Source: CAD feature listing. Evaluate the final solid. Frame: model axes, mm. A direction names the side the tool comes from. Round coordinates to 2 decimals unless told otherwise and drop trailing zeros. Write each loop counter-clockwise with the first axis right and the second up, starting at its lowest first coordinate (ties: lowest second). Pieces come first, ordered by that corner, then holes.
Autodesk Fusion 360 part; units mm, degrees
sketch "Sketch1" plane through (0, 0, 0) normal (0, 1, 0) x (1, 0, 0)
  line L0 (25, 18) -> (-25, 18) construction
  line L1 (-25, 18) -> (-25, -18) construction
  line L2 (-25, -18) -> (25, -18) construction
  line L3 (25, -18) -> (25, 18) construction
  line L4 (25, 18) -> (-25, -18) construction
  line L5 (-25, 18) -> (25, -18) construction
  arc A0 (25, 18) -> (-25, 18) centre (0, -84.6667) ccw
  arc A1 (-25, -18) -> (25, -18) centre (0, 84.6667) ccw
  arc A2 (25, -18) -> (25, 18) centre (-27.5, 0) ccw
  arc A3 (-25, 18) -> (-25, -18) centre (27.5, 0) ccw
  arc A4 (-23.0621, -15.8893) -> (23.0621, -15.8893) centre (0, 84.6667) ccw
  arc A5 (23.0621, -15.8893) -> (23.0621, 15.8893) centre (-27.5, 0) ccw
  arc A6 (23.0621, 15.8893) -> (-23.0621, 15.8893) centre (0, -84.6667) ccw
  arc A7 (-23.0621, 15.8893) -> (-23.0621, -15.8893) centre (27.5, 0) ccw
  dimension "d1" = 50
  dimension "d2" = 36
  dimension "d3" = 42
  dimension "d4" = 56
  dimension "d5" = 2.5
extrude "Extrude1" add sketch "Sketch1" along normal blind 170
sketch "Sketch3" plane through (0, 0, 0) normal (0, -1, 0) x (-1, 0, 0)
  arc A0 (23.0621, -15.8893) -> (23.0621, 15.8893) centre (-27.5, 0) ccw
  arc A1 (-23.0621, -15.8893) -> (23.0621, -15.8893) centre (0, 84.6667) ccw
  arc A2 (-23.0621, 15.8893) -> (-23.0621, -15.8893) centre (27.5, 0) ccw
  arc A3 (23.0621, 15.8893) -> (-23.0621, 15.8893) centre (0, -84.6667) ccw
  arc A4 (25, -18) -> (25, 18) centre (-27.5, 0) ccw
  arc A5 (25, 18) -> (-25, 18) centre (0, -84.6667) ccw
  arc A6 (-25, 18) -> (-25, -18) centre (27.5, 0) ccw
  arc A7 (-25, -18) -> (25, -18) centre (0, 84.6667) ccw
  line L0 (-23, -1) -> (23, -1)
  line L1 (23, -1) -> (23, 15)
  line L2 (23, 15) -> (-23, 15)
  line L3 (-23, 15) -> (-23, -1)
  line L4 (-23, -1) -> (23, 15) construction
  line L5 (23, -1) -> (-23, 15) construction
  arc A8 (23.0621, -15.8893) -> (23.0621, 15.8893) centre (-27.5, 0) ccw
  arc A9 (-23.0621, -15.8893) -> (23.0621, -15.8893) centre (0, 84.6667) ccw
  arc A10 (-23.0621, 15.8893) -> (-23.0621, -15.8893) centre (27.5, 0) ccw
  arc A11 (23.0621, 15.8893) -> (-23.0621, 15.8893) centre (0, -84.6667) ccw
  arc A12 (25, -18) -> (25, 18) centre (-27.5, 0) ccw
  arc A13 (25, 18) -> (-25, 18) centre (0, -84.6667) ccw
  arc A14 (-25, 18) -> (-25, -18) centre (27.5, 0) ccw
  arc A15 (-25, -18) -> (25, -18) centre (0, 84.6667) ccw
  arc A16 (23.0621, -15.8893) -> (23.0621, 15.8893) centre (-27.5, 0) ccw
  arc A17 (23.0621, 15.8893) -> (-23.0621, 15.8893) centre (0, -84.6667) ccw
  arc A18 (-23.0621, 15.8893) -> (-23.0621, -15.8893) centre (27.5, 0) ccw
  arc A19 (-23.0621, -15.8893) -> (23.0621, -15.8893) centre (0, 84.6667) ccw
  arc A20 (25, -18) -> (25, 18) centre (-27.5, 0) ccw
  arc A21 (-25, -18) -> (25, -18) centre (0, 84.6667) ccw
  arc A22 (-25, 18) -> (-25, -18) centre (27.5, 0) ccw
  arc A23 (25, 18) -> (-25, 18) centre (0, -84.6667) ccw
  line L6 (23, -1) -> (23, -8.5)
  line L7 (23, -8.5) -> (18, -8.5)
  line L8 (18, -8.5) -> (18, -16.9176)
  line L9 (-23, -1) -> (-23, -8.5)
  line L10 (-23, -8.5) -> (-18, -8.5)
  line L11 (-18, -8.5) -> (-18, -16.9176)
  dimension "d10" = 16
  dimension "d11" = 46
  dimension "d12" = 6
  dimension "d33" = 23.5
  dimension "d34" = 36
extrude "Extrude3" add sketch "Sketch3" against normal blind 170 contours A0 A1 A2 A3 L1 L2 L3 A8 A9 A10 A11 A16 A17 A18 A19 L6 L7 L8 L9 L10 L11
ref_plane "WorkPlane4" through (0, 150, 0) normal (0, 1, 0) x (0, 0, 1)
sketch "Sketch11" plane through (0, 150, 0) normal (0, 1, 0) x (1, 0, 0)
  line L0 (-18, -16.9176) -> (-18, -8.5)
  line L1 (-18, -8.5) -> (-23, -8.5)
  line L2 (-23, -8.5) -> (-23, 15)
  line L3 (-23, 15) -> (23, 15)
  line L4 (23, 15) -> (23, -8.5)
  line L5 (23, -8.5) -> (18, -8.5)
  line L6 (18, -8.5) -> (18, -16.9176)
  arc A0 (-18, -16.9176) -> (18, -16.9176) centre (0, 84.6667) ccw
  arc A1 (-25, 18) -> (-25, -18) centre (27.5, 0) ccw
  arc A2 (-25, -18) -> (25, -18) centre (0, 84.6667) ccw
  arc A3 (25, -18) -> (25, 18) centre (-27.5, 0) ccw
  arc A4 (25, 18) -> (-25, 18) centre (0, -84.6667) ccw
extrude "Extrude8" add sketch "Sketch11" along normal up to surface (20 mm away) contours L0 L1 L2 L3 L4 L5 L6 A0
sketch "Sketch8" plane through (0, 0, 0) normal (0, 0, 1) x (1, 0, 0)
  line L0 (-28, 170) -> (28, 160)
  line L1 (25, 0) -> (25, 170)
  line L2 (28, 160) -> (28, 210.2672)
  line L3 (28, 210.2672) -> (-28, 210.2672)
  line L4 (-28, 210.2672) -> (-28, 170)
  line L5 (28, 0) -> (25, 0)
  line L6 (-25, 0) -> (-28, 0)
  dimension "d35" = 160
  dimension "d36" = 170
extrude "Extrude7" cut sketch "Sketch8" along normal through all and the other way through all
ref_plane "WorkPlane3" through (-0.5274, 162.0467, 0) normal (0.1758, 0.9844, 0) x (-0.9844, 0.1758, 0)
sketch "Sketch12" plane through (0, 0, 0) normal (0, -1, 0) x (1, 0, 0)
  arc A0 (18, 16.9176) -> (-18, 16.9176) centre (0, -84.6667) ccw
  line L0 (18, 16.9176) -> (18, 8.5)
  line L1 (18, 8.5) -> (23, 8.5)
  line L2 (23, 8.5) -> (23, -15)
  line L3 (23, -15) -> (-23, -15)
  line L4 (-23, -15) -> (-23, 8.5)
  line L5 (-23, 8.5) -> (-18, 8.5)
  line L6 (-18, 8.5) -> (-18, 16.9176)
  arc A1 (-25, 18) -> (-25, -18) centre (27.5, 0) ccw
  arc A2 (-25, -18) -> (25, -18) centre (0, 84.6667) ccw
  arc A3 (25, -18) -> (25, 18) centre (-27.5, 0) ccw
  arc A4 (25, 18) -> (-25, 18) centre (0, -84.6667) ccw
extrude "Extrude9" cut sketch "Sketch12" along normal up to surface contours A0 L0 L1 L2 L3 L4 L5 L6 end surface through (-0.5274, 162.0467, 0) normal (0.175791, 0.984428, 0) offset 0
sketch "Sketch9" plane through (0, 0, 0) normal (0, -1, 0) x (1, 0, 0)
  arc A0 (18, 16.9176) -> (-18, 16.9176) centre (0, -84.6667) ccw
  line L0 (18, 16.9176) -> (18, 8.5)
  line L1 (18, 8.5) -> (23, 8.5)
  line L2 (23, 8.5) -> (23, -15)
  line L3 (23, -15) -> (-23, -15)
  line L4 (-23, -15) -> (-23, 8.5)
  line L5 (-23, 8.5) -> (-18, 8.5)
  line L6 (-18, 8.5) -> (-18, 16.9176)
  arc A1 (-25, 18) -> (-25, -18) centre (27.5, 0) ccw
  arc A2 (-25, -18) -> (25, -18) centre (0, 84.6667) ccw
  arc A3 (25, -18) -> (25, 18) centre (-27.5, 0) ccw
  arc A4 (25, 18) -> (-25, 18) centre (0, -84.6667) ccw
  line L7 (-33, 32.4232) -> (28, 32.4232)
  line L8 (28, 32.4232) -> (28, 15.5)
  line L9 (28, 15.5) -> (-33, 15.5)
  line L10 (-33, 15.5) -> (-33, 32.4232)
  dimension "d39" = 7
extrude "Extrude10" cut sketch "Sketch9" along normal up to surface contours A0 L0 L6 A1 A3 A4 L9 end surface through (-0.5274, 162.0467, 0) normal (0.175791, 0.984428, 0) offset 0
1) Section query B-B on z = -10. Return the cut outline in (x, y), then the cut area to 3 significant figures.
Taken from the geometry:
outline: (-27.09, 0) - (-23, 0) - (-23, 166.06) - (23, 157.85) - (23, 0) - (27.09, 0) - (27.09, 160.16) - (-27.09, 169.84) - close
area: 1,490 mm2
2) Section query D-D on z = 2. Return the cut outline in (x, y).
Taken from the geometry:
outline: (-27.96, 0) - (-23, 0) - (-23, 166.06) - (23, 157.85) - (23, 0) - (27.96, 0) - (27.96, 160.01) - (-27.96, 169.99) - close
3) Section query C-C on x = 21.5. Return the cut outline in (y, z), then the cut area to 3 significant figures.
Taken from the geometry:
outline: (0, -18.79) - (161.16, -18.79) - (161.16, 18.79) - (158.11, 18.79) - (158.11, 15.5) - (0, 15.5) - (0, 8.5) - (158.11, 8.5) - (158.11, -15) - (0, -15) - close
area: 1,820 mm2
4) Material intervals for line 1 (X direction, y = 32.5, z = 0.5); line 2 (X direction, y = 66.5, z = -13); line 3 (Z direction, x = -21.5, y = 21), sorted ascending.
Taken from the geometry:
line 1: x = -28 to -23, 23 to 28
line 2: x = -26.46 to -23, 23 to 26.46
line 3: z = -18.79 to -15, 8.5 to 15.5
5) Reachability of faces 1 (the face through (-23, 82, -3)), 2 (the face through (-27.87, 83.81, -3.81)), 3 (the face through (18, 78, 12)), 4 (the face through (22, 78, 15.5)) from +Z, -Z, +X, -X, +Y, -Y: full face, straight path, thin tool, end or side. Return the list, or none.
Taken from the geometry:
face 1: -Y
face 2: -X, +Y, -Y
face 3: +Z, -Y
face 4: +Z, +X, -X, -Y
6) Section query A-A on y = 31. Return the cut outline in (x, z), then the cut area to 3 significant figures.
Taken from the geometry:
outline: (-25.79, 15.5) arc R55.5 ccw to (-25, -18) arc R105.67 ccw to (25, -18) arc R55.5 ccw to (25.79, 15.5) - (18, 15.5) - (18, 8.5) - (23, 8.5) - (23, -15) - (-23, -15) - (-23, 8.5) - (-18, 8.5) - (-18, 15.5) - close
area: 585 mm2
7) Pull-direction query (Z, two-part tool) for faces 5 (the face through (21, 78, 8.5)), 6 (the face through (0, 84, -21)), 7 (the face through (-0.4, 0, -15.2)), 8 (the face through (-22, 82, 15.5)); classes: released by +Z, released by -Z, zero draft, split by the parting line, or undercut.
Taken from the geometry:
face 5: undercut
face 6: released by -Z
face 7: zero draft
face 8: released by +Z
8) Contact query for flat-ended pins moving along their axis: P1, Ø6, axis at x = -9, z = -6, coming from the -Y side; P2, Ø2, axis at y = 66, z = -7, coming from the +X side; P3, Ø3, axis at y = 20, z = -10.5, coming from the -X side. Output: stop coordinate, or through.
Taken from the geometry:
P1: stops at y = 163.02
P2: stops at x = 27.67
P3: stops at x = -27.27
